Autodesk Inventor part; units mm, degrees
ref_plane "YZ Plane" through (0, 0, 0) normal (1, 0, 0) x (0, 1, 0)
ref_plane "XZ Plane" through (0, 0, 0) normal (0, 1, 0) x (-1, 0, 0)
ref_plane "XY Plane" through (0, 0, 0) normal (0, 0, 1) x (1, 0, 0)
sketch "草图1" plane through (0, 0, 0) normal (0, 1, 0) x (-1, 0, 0)
  line L0 (20, 9) -> (-20, 9)
  line L1 (-20, 9) -> (-20, -9)
  line L2 (-20, -9) -> (20, -9)
  line L3 (20, 5.1) -> (12.5, 3.2)
  line L4 (12.5, 3.2) -> (5, 5.2)
  line L5 (5, 0) -> (0, 0)
  line L6 (20, -5.1) -> (12.5, -3.2)
  line L7 (12.5, -3.2) -> (5, -5.2)
  line L8 (-13, 9) -> (-13, -9)
  line L9 (20, -9) -> (20, -5.1)
  line L10 (20, 5.1) -> (20, 9)
  line L11 (5, 5.2) -> (5, -5.2)
  line L12 (5, -5.2) -> (-20, -5.2)
  line L13 (-12.9, 9) -> (-12.9, -2)
  line L14 (-12.9, -2) -> (-16, -2)
  line L15 (-16, -2) -> (-16, 9)
  line L16 (-12.9, -2) -> (-16, -2)
  line L17 (-16, -2) -> (-16, 9)
  line L18 (-16, 9) -> (-12.9, 9)
  line L19 (-12.9, 9) -> (-12.9, -2)
  dimension "d0" = 18
  dimension "d1" = 40
  dimension "d4" = 3.9
  dimension "d6" = 5.8
  dimension "d8" = 3.8
  dimension "d13" = 33
  dimension "d14" = 11
  dimension "d15" = 3.1
  dimension "d16" = 4
  dimension "d39" = 9
extrude "拉伸1" add sketch "草图1" along normal blind 50
extrude "拉伸2" cut sketch "草图1" along normal blind 50 contours L13 L14 L8 L0 | L8 L14 L15 L0
sketch "草图2" plane through (20, 0, 9) normal (0, 0, 1) x (1, 0, 0)
  line L0 (-4, 50) -> (-4, 0)
  line L1 (-4, 0) -> (0, 0)
  line L2 (0, 0) -> (0, 50)
  line L3 (-4, 50) -> (0, 50)
  line L4 (-4, 50) -> (-4, 0)
  line L5 (0, 0) -> (0, 50)
  line L6 (-4, 8.5) -> (0, 8.5)
  line L7 (0, 8.5) -> (0, 41.5)
  line L8 (0, 41.5) -> (-4, 41.5)
  line L9 (-4, 41.5) -> (-4, 8.5)
  point P0 (-20, 0)
  point P1 (-4, 25)
  dimension "d19" = 33
extrude "拉伸3" cut sketch "草图2" against normal up to next contours L3 L2 L8 L0 | L6 L2 L1 L0
chamfer "倒角1" distance 2 distance2 8 1 edges at (16, 0, -5.5) measured on face at (6.9333, 0, 4.0667)
chamfer "倒角2" distance 2 distance2 8 1 edges at (16, 50, -5.5) measured on face at (6.9333, 50, 4.0667)
sketch "草图3" plane through (-20, 0, 9) normal (0, 0, 1) x (1, 0, 0)
  line L0 (15, 0) -> (15, 50)
  line L1 (15, 0) -> (15, 50)
  line L2 (32.9, 0) -> (32.9, 50)
  line L3 (11.9, 20.5) -> (27.9, 20.5)
  line L4 (27.9, 20.5) -> (27.9, 41.5)
  line L5 (27.9, 41.5) -> (11.9, 41.5)
  line L6 (11.9, 41.5) -> (11.9, 20.5)
  line L7 (0, 50) -> (32.9, 50)
  line L8 (20, 5) -> (27.9, 5)
  line L9 (27.9, 5) -> (27.9, 15.5)
  line L10 (27.9, 15.5) -> (20, 15.5)
  line L11 (20, 15.5) -> (20, 5)
  line L12 (0, 0) -> (32.9, 0)
  point P0 (20, 0)
  dimension "d28" = 21
  dimension "d29" = 8.5
  dimension "d30" = 5
  dimension "d32" = 21
  dimension "d35" = 5
  dimension "d36" = 5
  dimension "d37" = 5
  dimension "d38" = 5
extrude "拉伸4" cut sketch "草图3" against normal blind 50 contours L3 L6 L5 L0 | L0 L5 L4 L3 | L11 L10 L9 L8
sketch "草图4" plane through (-20, 0, 9) normal (0, 0, 1) x (1, 0, 0)
  line L0 (27.9, 15.5) -> (27.9, 5)
  line L1 (27.9, 5) -> (20, 5)
  line L2 (20, 5) -> (20, 15.5)
  line L3 (20, 15.5) -> (27.9, 15.5)
  line L4 (27.9, 41.5) -> (27.9, 20.5)
  line L5 (27.9, 20.5) -> (11.9, 20.5)
  line L6 (11.9, 20.5) -> (11.9, 41.5)
  line L7 (11.9, 41.5) -> (27.9, 41.5)
  line L8 (32.9, 0) -> (32.9, 50)
  line L9 (0, 50) -> (32.9, 50)
  line L10 (0, 0) -> (0, 50)
  line L11 (0, 0) -> (32.9, 0)
  line L12 (36, 8.5) -> (40, 8.5)
  line L13 (40, 8.5) -> (40, 41.5)
  line L14 (40, 41.5) -> (36, 41.5)
  line L15 (36, 41.5) -> (36, 8.5)
  point P0 (20, 0)
extrude "拉伸6" add sketch "草图4" along normal blind 2 contours L15 L14 L13 L12
properties part number "latte_d435_frame_new_legs"
Part model, mm, in its own coordinate system. A direction names the side the tool comes from. Coordinates: 2 decimals unless noted, no trailing zeros. Loops run counter-clockwise (first coordinate to the right, second up) from the corner with the lowest first, then second, coordinate; pieces in that order, holes last. Notation, with made-up numbers: (-19, 71.25) - (23, 71.25) arc R22 ccw to (23, 110.25) - close; hole circle Ø2 at (23.5, -28.5). An arc over 180 degrees is marked (long way). Write item = value, one per line. Start each with the question number.
Item 1: Flat gauge pins, fed straight in: pin 1 Ø0.6 at (y, z) = (42, -4.5) entering from +X; pin 2 Ø4 at (y, z) = (47.5, -0.5) entering from -X; pin 3 Ø10 at (x, y) = (1.5, 14) entering from +Z. Where does each tip first touch, or does it go through?
Item 2: Cut at D-D, the plane x = -3. Give the cut face in (y, z), and give its area (3 significant figures).
Item 3: Cut at B-B, the plane y = 12. Give the cut face in (x, z).
Item 4: Wall check: L1, parallel to X at y = 35, z = 8.5; L2, parallel to Y at x = 6, z = 8.75; L3, parallel to X at y = 6, z = -2.75. Give the ranges that are in metal, low to high. Write a range as from..to.
Item 5: Cut at A-A, the plane x = -15.5. Give the cut face in (y, z).
Item 6: Mould opens along Z. For faces 1 (the flat face through (20, 25, 1)), 2 (the flat face through (18, 25, 11)), 3 (the flat face through (-16.302, 24.65, -4.163)) say: released by +Z, released by -Z, zero draft, split by the parting line, or undercut.
Item 7: Cut at C-C, the plane y = 32.5. Give the cut face in (x, z), and give its area (3 significant figures).
Item 8: 3-axis set-ups, long thin cutter, end or side, ignore diameter. For faces 4 (the flat face through (16, 25, 4)), 5 (the flat face through (18, 8.5, 1)), 6 (the flat face through (-5, 10, 0)), 7 (the flat face through (7.9, 31, 0)): which of +Z, -Z, +X, -X, +Y, -Y reach the whole face in a straight line?
The answers:
q1.pin_1 = 16
q1.pin_2 = -5
q1.pin_3 = 9
q2.outline = (0, -9) - (20.5, -9) - (20.5, 9) - (0, 9) - close; (41.5, -9) - (50, -9) - (50, 9) - (41.5, 9) - close
q2.area = 522 mm2
q3.outline = (-20, -9) - (0, -9) - (0, 9) - (-20, 9) - (-20, 5.1) - (-12.5, 3.2) - (-5, 5.2) - (-5, -5.2) - (-12.5, -3.2) - (-20, -5.1) - close; (7.9, -9) - (20, -9) - (20, 11) - (16, 11) - (16, -2) - (12.9, -2) - (12.9, 9) - (7.9, 9) - close
q4.L1 = -20..-8.1, 7.9..12.9, 16..20
q4.L2 = 0..5, 15.5..20.5, 41.5..50
q4.L3 = -5..0, 7.9..15.5
q5.outline = (0, -9) - (50, -9) - (50, -3.96) - (0, -3.96) - close; (0, 3.96) - (50, 3.96) - (50, 9) - (0, 9) - close
q6.face_1 = zero draft
q6.face_2 = released by +Z
q6.face_3 = undercut
q7.outline = (-20, -9) - (-8.1, -9) - (-8.1, -4.37) - (-12.5, -3.2) - (-20, -5.1) - close; (-20, 5.1) - (-12.5, 3.2) - (-8.1, 4.37) - (-8.1, 9) - (-20, 9) - close; (7.9, -9) - (20, -9) - (20, 11) - (16, 11) - (16, -2) - (12.9, -2) - (12.9, 9) - (7.9, 9) - close
q7.area = 310 mm2
q8.face_4 = +Z, +Y, -Y
q8.face_5 = +Z, -Z, +X, -Y
q8.face_6 = +Y, -Y
q8.face_7 = +Z, -Z
